```python
from build123d import *

# Parameters (mm, degrees)
EXTRUDE_1_DEPTH     = 12
SKETCH_2_R          = 5.5
CUT_EXTRUDE_1_DEPTH = 38.107950631


with BuildPart() as part:
    # 草图1 → 凸台-拉伸1 (new, symmetric)
    with BuildSketch(Plane.XY):
        with BuildLine():
            Line((-33, 0), (-33, 8))
            Line((-33, 8), (-18.33030278, 8))
            ThreePointArc((-18.33030278, 8), (0, 20), (18.33030278, 8))
            Line((18.33030278, 8), (33, 8))
            Line((33, 8), (33, 0))
            Line((33, 0), (13, 0))
            ThreePointArc((13, 0), (0, 13), (-13, 0))
            Line((-13, 0), (-33, 0))
        make_face()
    extrude(amount=EXTRUDE_1_DEPTH, both=True)

    # 草图2 → 切除-拉伸1 (cut, through all)
    with BuildSketch(Plane(origin=(0, 8, 0), x_dir=(1, 0, 0), z_dir=(0, 1, 0))):
        with Locations(Location((25, 0, 0), (0, 0, 180))):
            Circle(SKETCH_2_R)
        with Locations((-25, 0)):
            Circle(SKETCH_2_R)
    extrude(amount=-CUT_EXTRUDE_1_DEPTH, mode=Mode.SUBTRACT)


solid = part.part
```
Geometry check sheet. Reference: the model listing, model coordinates, mm. A direction names the side the tool comes from. Coordinates: 2 decimals unless noted, no trailing zeros. Order: outer loops, then holes, each group sorted by start corner. A loop starts at its lowest first (then second) coordinate and runs counter-clockwise, first axis right, second up.
Item 1: Mould release check, pull along X, two halves, no side actions. Record for faces 3 (the flat face through (-31, 8, 0)), 4 (the cylindrical face through (0, 13, 0)), 5 (the flat face through (33, 4, 0)): released by +X, released by -X, zero draft, split by the parting line, or undercut.
Item 2: Section check C-C (y = 6.5). Enter the section's corners in (x, z), plus the area to 3 significant figures.
Item 3: Section check A-A (x = -25). Enter the section's corners in (y, z).
Item 4: Section check D-D (z = 9.25). Enter the section's corners in (x, y), plus the area to 3 significant figures.
Item 5: Tool access check on faces 1 (the flat face through (26, 8, 6)), 2 (the cylindrical face through (0, 20, 0)). Record the directions out of +Z, -Z, +X, -X, +Y, -Y that give a thin tool (end or side, any length) a straight path to the whole face; none if there is none.
Item 6: Depth check by flat-ended pin: pin 1 (7.5 mm diameter, centred on x = -24, z = 3.5, fed in from +Y); pin 2 (2 mm diameter, centred on x = 0.5, z = -0.5, fed in from -Y); pin 3 (5 mm diameter, centred on x = -9.5, z = 6.5, fed in from -Y). Enter the tip coordinate at first touch or a pass-through.
Item 7: Scan lines: line 1 along Z through (x, y) = (25, 3); line 2 along X through (y, z) = (5.5, -1.5); line 3 along X through (y, z) = (5, 1.25). Record each from-to range of solid material in increasing order.
Item 8: Section check B-B (z = 0). Enter the section's corners in (x, y), plus the area to 3 significant figures.
Check sheet entries:
1. face 3: zero draft
1. face 4: undercut
1. face 5: released by +X
2. outline: (-33, -12) - (-11.26, -12) - (-11.26, 12) - (-33, 12) - close; (11.26, -12) - (33, -12) - (33, 12) - (11.26, 12) - close; hole circle Ø11 at (-25, 0); hole circle Ø11 at (25, 0)
2. area: 854 mm2
3. outline: (0, -12) - (8, -12) - (8, -5.5) - (0, -5.5) - close; (0, 5.5) - (8, 5.5) - (8, 12) - (0, 12) - close
4. outline: (-33, 0) - (-13, 0) arc R13 cw to (13, 0) - (33, 0) - (33, 8) - (18.33, 8) arc R20 ccw to (-18.33, 8) - (-33, 8) - close
4. area: 580 mm2
5. face 1: +Z, -Z, +X, +Y
5. face 2: +Z, -Z, +Y
6. pin 1: stops at y = 8
6. pin 2: stops at y = 12.91
6. pin 3: stops at y = 5
7. line 1: z = -12 to -5.5, 5.5 to 12
7. line 2: x = -33 to -30.29, -19.71 to -11.78, 11.78 to 19.71, 30.29 to 33
7. line 3: x = -33 to -30.36, -19.64 to -12, 12 to 19.64, 30.36 to 33
8. outline: (-33, 0) - (-30.5, 0) - (-30.5, 8) - (-33, 8) - close; (-19.5, 0) - (-13, 0) arc R13 cw to (13, 0) - (19.5, 0) - (19.5, 8) - (18.33, 8) arc R20 ccw to (-18.33, 8) - (-19.5, 8) - close; (30.5, 0) - (33, 0) - (33, 8) - (30.5, 8) - close
8. area: 404 mm2
